Input: part model. Units: mm. Frame: model coordinates. A direction names the side the tool comes from. Coordinates: 2 decimals unless noted, no trailing zeros. Loops run counter-clockwise (first coordinate to the right, second up) from the corner with the lowest first, then second, coordinate; pieces in that order, holes last. Notation, with made-up numbers: (55.5, -35.75) -> (79.5, -35.75) arc R15 cw to (79.5, -17.75) -> close; hole circle Ø1 at (2, 76.5). An arc over 180 degrees is marked (long way). Put each result on its own line as item: value. Start each with the question number.
1) Material intervals for L1, parallel to Y at x = 5, z = 47; L2, parallel to X at y = -12, z = 14, sorted ascending.
2) Cut plane A-A (y = 0). Return the cut outline in (x, z).
3) Contact query for flat-ended pins moving along their axis: P1, Ø16, axis at x = 1.5, z = 21.5, coming from the +Y side; P2, Ø5, axis at x = 14, z = 30, coming from the -Y side; P3, Ø6, axis at x = 3, z = 19.5, coming from the -Y side. Output: stop coordinate, or through.
4) Cut plane B-B (z = 18). Return the cut outline in (x, y).
5) Cut plane D-D (z = 52.5). Return the cut outline in (x, y), plus the area to 3 significant figures.
6) Cut plane C-C (x = 20.5). Return the cut outline in (y, z), plus the area to 3 significant figures.
7) Pull-direction query (Y, two-part tool) for faces 1 (the flat face through (0, 10, 35)), 2 (the flat face through (10, -15, 23)), 3 (the cylindrical face through (27.26, -13.39, 40.55)); classes: pulls with the +Y half, pulls with the -Y half, needs draft (parallel to the pull), parting line crosses it, or undercut.
8) Set-up query: faces 4 (the flat face through (10, 15, 23)), 5 (the flat face through (10, -0.1, 0.9)), 6 (the flat face through (0, -10, 35)). Return all of +Z, -Z, +X, -X, +Y, -Y with unobstructed straight access to the full face (end or side cutting, diameter ignored); none if empty.
from build123d import *

# Parameters (mm, degrees)
SKIZZE3_W                       = 20
SKIZZE3_H                       = 20
AUFSATZ_LINEAR_AUSTRAGEN2_DEPTH = 70
SKIZZE4_R                       = 22
AUFSATZ_LINEAR_AUSTRAGEN3_DEPTH = 35


with BuildPart() as part:
    # Skizze3 → Aufsatz-Linear austragen2 (new body)
    with BuildSketch(Plane.XY):
        Rectangle(SKIZZE3_W, SKIZZE3_H)
    extrude(amount=AUFSATZ_LINEAR_AUSTRAGEN2_DEPTH)

    # Skizze4 → Aufsatz-Linear austragen3 (add)
    with BuildSketch(Plane(origin=(10, 0, 0), x_dir=(0, 0, -1), z_dir=(1, 0, 0))):
        with Locations((-23.092221055, 0)):
            Circle(SKIZZE4_R)
    extrude(amount=AUFSATZ_LINEAR_AUSTRAGEN3_DEPTH)


solid = part.part
Results found:
1. L1: y = -10 to 10
1. L2: x = 10 to 45
2. outline: (-10, 0) -> (10, 0) -> (10, 1.09) -> (45, 1.09) -> (45, 45.09) -> (10, 45.09) -> (10, 70) -> (-10, 70) -> close
3. P1: stops at y = 10
3. P2: stops at y = -21.55
3. P3: stops at y = -10
4. outline: (-10, -10) -> (10, -10) -> (10, -21.4) -> (45, -21.4) -> (45, 21.4) -> (10, 21.4) -> (10, 10) -> (-10, 10) -> close
5. outline: (-10, -10) -> (10, -10) -> (10, 10) -> (-10, 10) -> close
5. area: 400 mm2
6. outline: circle Ø44 at (0, 23.09)
6. area: 1,520 mm2
7. face 1: pulls with the +Y half
7. face 2: needs draft
7. face 3: parting line crosses it
8. face 4: +Z, -Z, -X, +Y
8. face 5: -Z, +X
8. face 6: +Z, -Z, -X, -Y
